```python
from build123d import *

# Parameters (mm, degrees)
F0_R       = 10
F1_DEPTH   = 4
F2_R       = 4.85
F3_DEPTH   = 3.5
F4_R       = 6.95
F4_R_2     = 6
F5_DEPTH   = 0.5
F6_R       = 10
F6_R_2     = 6.95
F7_DEPTH   = 3
F8_SIZE    = 0.25
F9_SIZE2   = 0.99999
F9_SIZE    = 0.49999
F9_2_SIZE2 = 1
F9_2_SIZE  = 0.5
F10_R      = 12.5
F10_R_2    = 9.5
F11_DEPTH  = 0.2


# Not quite as in the source:
# - a fillet or chamfer is up to 0.001 mm smaller than in the source, because OpenCascade refuses the exact size


with BuildPart() as f1:
    # F0 (on Right) → F1 (new body)
    with BuildSketch(Plane.YZ):
        Circle(F0_R)
    extrude(amount=F1_DEPTH)

    # F2 (on face) → F3 (join)
    with BuildSketch(Plane(origin=(0, 0, 0), x_dir=(0, -1, 0), z_dir=(-1, 0, 0))):
        Circle(F2_R)
    extrude(amount=F3_DEPTH)

    # F4 (on face) → F5 (join)
    with BuildSketch(Plane(origin=(0, 0, 0), x_dir=(0, -1, 0), z_dir=(-1, 0, 0))):
        Circle(F4_R)
        Circle(F4_R_2, mode=Mode.SUBTRACT)
    extrude(amount=F5_DEPTH)

    # F6 (on face) → F7 (cut)
    with BuildSketch(Plane(origin=(0, 0, 0), x_dir=(0, -1, 0), z_dir=(-1, 0, 0))):
        Circle(F6_R)
        Circle(F6_R_2, mode=Mode.SUBTRACT)
    extrude(amount=-F7_DEPTH, mode=Mode.SUBTRACT)

    # F8
    f8_edges = [f1.edges().sort_by_distance(p)[0] for p in [
        (-0.5, 6.95, 0),
        (-0.5, 6, 0),
    ]]
    chamfer(f8_edges, length=F8_SIZE)

    # F9 (size 0.5 and 1 in the source; OpenCascade refuses exactly that, so slightly less here)
    f9_edges = [f1.edges().sort_by_distance(p)[0] for p in [
        (4, -10, 0),
    ]]
    f9_side = f1.faces().sort_by_distance((4, 0, 0))[0]
    chamfer(f9_edges, length=F9_SIZE, length2=F9_SIZE2, reference=f9_side)

    # F9#2
    f9_2_edges = [f1.edges().sort_by_distance(p)[0] for p in [
        (-3.5, 4.85, 0),
    ]]
    f9_2_side = f1.faces().sort_by_distance((-3.5, 0, 0))[0]
    chamfer(f9_2_edges, length=F9_2_SIZE, length2=F9_2_SIZE2, reference=f9_2_side)

    # F10 (on face) → F11 (join)
    with BuildSketch(Plane.YZ.offset(4)):
        Circle(F10_R)
        Circle(F10_R_2, mode=Mode.SUBTRACT)
    extrude(amount=-F11_DEPTH)


solid = f1.part
```
Source: CAD feature listing. Evaluate the final solid. Frame: model axes, mm. A direction names the side the tool comes from. Coordinates: 2 decimals unless noted, no trailing zeros. Loops run counter-clockwise (first coordinate to the right, second up) from the corner with the lowest first, then second, coordinate; pieces in that order, holes last. Notation, with made-up numbers: (48, -9.5) - (105, -9.5) arc R23 ccw to (105, 4.5) - close; hole circle Ø5 at (61, -12.5). An arc over 180 degrees is marked (long way). Answer as CSV lines item,"result".
1. Ray query, line 1 (Z direction, x = -0.2, y = 0); line 2 (X direction, y = -8.75, z = 3.25); line 3 (X direction, y = 5.5, z = 10.75). Return the intervals inside material, ascending.
Established:
line 1,"z = -6.95 to -6, -4.85 to 4.85, 6 to 6.95"
line 2,"x = 3 to 4"
line 3,"x = 3.8 to 4"
2. Section B-B (x = -3). Return loops of the section in (y, z), then the cut area to 3 significant figures.
Established:
outline,"circle Ø9.2 at (0, 0)"
area,"66.5 mm2"
3. Section C-C (x = 0.5). Return loops of the section in (y, z), then the cut area to 3 significant figures.
Established:
outline,"circle Ø13.9 at (0, 0)"
area,"152 mm2"
4. Reachability of faces 4 (the flat face through (4, 0, 0)), 5 (the cylindrical face through (-1.232, -4.626, 1.457)) from +Z, -Z, +X, -X, +Y, -Y: full face, straight path, thin tool, end or side. Return the list, or none.
Established:
face 4,"+Z, -Z, +X, +Y, -Y"
face 5,"-X"
5. Contact query for flat-ended pins moving along their axis: pin 1 (4 mm diameter, centred on y = 1.5, z = -8, fed in from -X); pin 2 (10 mm diameter, centred on y = -4.5, z = 1, fed in from -X); pin 3 (1 mm diameter, centred on x = 1, y = 7.5, fed in from -Z); pin 4 (3 mm diameter, centred on x = 0.5, z = 7.5, fed in from +Y). Output: stop coordinate, or through.
Established:
pin 1,"stops at x = -0.5"
pin 2,"stops at x = -3.5"
pin 3,"passes through"
pin 4,"stops at y = 3.51"
6. Mould query, pull axis Z, two halves, no side actions, for faces 1 (the flat face through (0, 5, 0)), 2 (the flat face through (3, -2, 7)), 3 (the cylindrical face through (1.352, 1.507, -6.785)). Classes: released by +Z, released by -Z, zero draft, split by the parting line, or undercut.
Established:
face 1,"undercut"
face 2,"zero draft"
face 3,"split by the parting line"
